Model file for the job. Use its own axes, mm. Face numbers are marked on the shaded views. A direction names the side the tool comes from. Give positions to 0.01 mm unless a question says otherwise; leave off trailing zeros. Order: outer loops, then holes, each group sorted by start corner. A loop starts at its lowest first (then second) coordinate and runs counter-clockwise, first axis right, second up. Notation, with made-up numbers: M 45.5,76 L 52.5,76 A20 cw 52.5,110 Z; hole C 62.5,8.25 d10. An arc over 180 degrees is marked long. Return JSON: item names as keys, results as strings. Group by question number.
1. Slice it at C-C on z = -0.75. List the corners of the cut face in (x, y), then the cut area to 3 significant figures.
2. Pin check, flat tips, straight feed: pin 1 (1 mm diameter, centred on y = 0, z = -5, fed in from +X); pin 2 (1.5 mm diameter, centred on x = 2.5, y = 2.5, fed in from -Z); pin 3 (4 mm diameter, centred on x = -1.5, z = -1, fed in from +Y); pin 4 (2 mm diameter, centred on y = 1.5, z = -5, fed in from +X). Stop position of each tip, or through.
3. Slice it at B-B on z = -4.5. List the corners of the cut face in (x, y).
4. Slice it at A-A on x = 0. List the corners of the cut face in (y, z).
5. 3-axis set-ups, long thin cutter, end or side, ignore diameter. For the marked faces 1 and 2: which of +Z, -Z, +X, -X, +Y, -Y reach the whole face in a straight line?
6. Wall check: probe 1 along Y at (x, z) = (0, -3); probe 2 along Y at (x, z) = (0.75, 0.25); probe 3 along Z at (x, y) = (2, -2.5). Give the ranges that are in metal, low to high. Write a range as [from, to].
from build123d import *

# Parameters (mm, degrees)
SKETCH_1_R          = 3.5
SKETCH_1_R_2        = 2.75
SKETCH_1_R_3        = 2.25
EXTRUDE_1_DEPTH     = 0.3
SKETCH_1_4_R        = 2.75
SKETCH_1_4_R_2      = 2.25
EXTRUDE_2_DEPTH     = 6.5
CUT_EXTRUDE_1_DEPTH = 2.7
FILLET_1_R          = 0.05


with BuildPart() as part:
    # Sketch 1 → Extrude 1 (new body)
    with BuildSketch(Plane.XY):
        Circle(SKETCH_1_R)
        Circle(SKETCH_1_R_2, mode=Mode.SUBTRACT)
        Circle(SKETCH_1_R_2)
        Circle(SKETCH_1_R_3, mode=Mode.SUBTRACT)
    extrude(amount=EXTRUDE_1_DEPTH)

    # Sketch 1_4 → Extrude 2 (add)
    with BuildSketch(Plane.XY):
        Circle(SKETCH_1_4_R)
        Circle(SKETCH_1_4_R_2, mode=Mode.SUBTRACT)
    extrude(amount=-EXTRUDE_2_DEPTH)

    # Sketch 2 → Cut-Extrude 1 (cut)
    with BuildSketch(Plane(origin=(0, 0, -6.5), x_dir=(-1, 0, 0), z_dir=(0, 0, -1))):
        with BuildLine():
            ThreePointArc((-0.65, 2.672077843), (-2.75, 0), (-0.65, -2.672077843))
            Line((-0.65, -2.672077843), (-0.65, -2.154065923))
            ThreePointArc((-0.65, -2.154065923), (-2.25, 0), (-0.65, 2.154065923))
            Line((-0.65, 2.154065923), (-0.65, 2.672077843))
        make_face()
        with BuildLine():
            Line((0.65, -2.154065923), (0.65, -2.672077843))
            ThreePointArc((0.65, -2.672077843), (2.162174831, -1.699264547), (2.75, 0))
            ThreePointArc((2.75, 0), (2.162174831, 1.699264547), (0.65, 2.672077843))
            Line((0.65, 2.672077843), (0.65, 2.154065923))
            ThreePointArc((0.65, 2.154065923), (1.806239187, 1.341640786), (2.25, 0))
            ThreePointArc((2.25, 0), (1.806239187, -1.341640786), (0.65, -2.154065923))
        make_face()
    extrude(amount=-CUT_EXTRUDE_1_DEPTH, mode=Mode.SUBTRACT)

    # Fillet 1
    fillet_1_edges = [part.edges().sort_by_distance(p)[0] for p in [
        (2.162174831, -1.699264547, -3.8),
        (0.65, -2.413071883, -6.5),
        (0.65, 2.413071883, -6.5),
        (0, -2.75, -6.5),
        (0, -2.25, -6.5),
        (-0.65, -2.413071883, -6.5),
        (-0.65, 2.413071883, -6.5),
        (-2.75, 0, -3.8),
        (-3.5, 0, 0),
        (-3.5, 0, 0.3),
        (0, 2.75, -6.5),
        (0, 2.25, -6.5),
    ]]
    fillet(fillet_1_edges, radius=FILLET_1_R)


solid = part.part
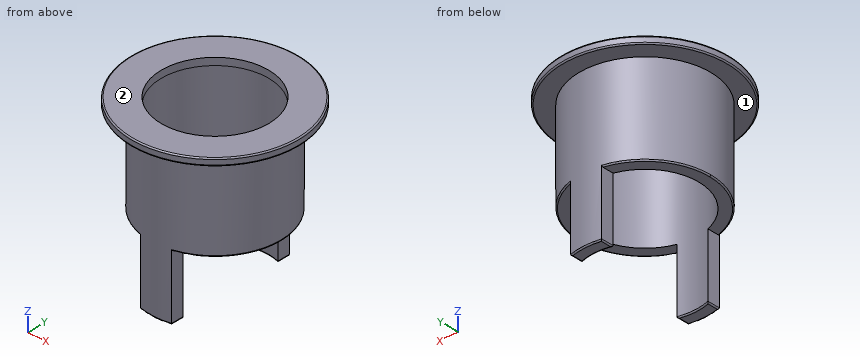
Result:
{
 "1": {"outline": "C 0,0 d5.5; hole C 0,0 d4.5", "area": "7.85 mm2"},
 "2": {"pin 1": "passes through", "pin 2": "stops at z = 0", "pin 3": "stops at y = 3.5", "pin 4": "stops at x = 0.65"},
 "3": {"outline": "M -0.65,-2.67 A2.75 ccw 0.65,-2.67 L 0.65,-2.15 A2.25 cw -0.65,-2.15 Z; M -0.65,2.15 A2.25 cw 0.65,2.15 L 0.65,2.67 A2.75 ccw -0.65,2.67 Z"},
 "4": {"outline": "M -3.5,0.05 A0.05 ccw -3.45,0 L -2.75,0 L -2.75,-6.45 A0.05 ccw -2.7,-6.5 L -2.3,-6.5 A0.05 ccw -2.25,-6.45 L -2.25,0.3 L -3.45,0.3 A0.05 ccw -3.5,0.25 Z; M 2.25,-6.45 A0.05 ccw 2.3,-6.5 L 2.7,-6.5 A0.05 ccw 2.75,-6.45 L 2.75,0 L 3.45,0 A0.05 ccw 3.5,0.05 L 3.5,0.25 A0.05 ccw 3.45,0.3 L 2.25,0.3 Z"},
 "5": {"face 1": "-Z", "face 2": "+Z, +X, -X, +Y, -Y"},
 "6": {"probe 1": "y = [-2.75, -2.25], [2.25, 2.75]", "probe 2": "y = [-3.42, -2.12], [2.12, 3.42]", "probe 3": "z = [0, 0.3]"}
}
